Could you check a few things on this model? Use its own coordinates, in mm. A direction names the side the tool comes from. Give positions to 0.01 mm unless a question says otherwise; leave off trailing zeros. Order: outer loops, then holes, each group sorted by start corner. A loop starts at its lowest first (then second) coordinate and runs counter-clockwise, first axis right, second up. Notation, with made-up numbers: (-10, 72.25) -> (24, 72.25) arc R19 ccw to (24, 83.25) -> close; hole circle Ø8 at (-35.5, -7.75). An arc over 180 degrees is marked (long way). Write each question's results on one line, items separated by ' | '.
```python
from build123d import *

# Parameters (mm, degrees)
SKETCH1_R           = 3.6
BOSS_EXTRUDE2_DEPTH = 6
SKETCH4_R           = 4.250000009
BOSS_EXTRUDE3_DEPTH = 9
SKETCH7_R           = 2.1082
CUT_EXTRUDE3_DEPTH  = 5.6
SKETCH5_R           = 2.000000064
BOSS_EXTRUDE6_DEPTH = 9.156
FILLET3_R           = 0.7
SKETCH9_R           = 3.000000096
BOSS_EXTRUDE7_DEPTH = 5.6
FILLET4_R           = 0.7


with BuildPart() as part:
    # Sketch1 → Boss-Extrude2 (new body)
    with BuildSketch(Plane(origin=(0, 0, 0), x_dir=(1, 0, 0), z_dir=(0, 1, 0))):
        with Locations(Location((0, 0, 0), (0, 0, 270))):
            Circle(SKETCH1_R)
    extrude(amount=BOSS_EXTRUDE2_DEPTH)

    # Sketch4 → Boss-Extrude3 (add)
    with BuildSketch(Plane(origin=(0, 0, 0), x_dir=(1, 0, 0), z_dir=(0, 1, 0))):
        with Locations(Location((0, 0, 0), (0, 0, 270))):
            Circle(SKETCH4_R)
    extrude(amount=-BOSS_EXTRUDE3_DEPTH)

    # Sketch7 → Cut-Extrude3 (cut)
    with BuildSketch(Plane(origin=(0, 6, 0), x_dir=(1, 0, 0), z_dir=(0, 1, 0))):
        with Locations(Location((0, 0, 0), (0, 0, 270))):
            Circle(SKETCH7_R)
    extrude(amount=-CUT_EXTRUDE3_DEPTH, mode=Mode.SUBTRACT)

    # Sketch5 → Boss-Extrude6 (add)
    with BuildSketch(Plane(origin=(0, 0, 0), x_dir=(1, 0, 0), z_dir=(0, 1, 0))):
        with Locations(Location((0, 0, 0), (0, 0, 270))):
            Circle(SKETCH5_R)
    extrude(amount=BOSS_EXTRUDE6_DEPTH)

    # Fillet3
    fillet3_edges = [part.edges().sort_by_distance(p)[0] for p in [
        (0, 6, -2.1082),
        (0, 6, -3.6),
    ]]
    fillet(fillet3_edges, radius=FILLET3_R)

    # Sketch9 → Boss-Extrude7 (add)
    with BuildSketch(Plane(origin=(0, 9.156, 0), x_dir=(1, 0, 0), z_dir=(0, 1, 0))):
        with Locations(Location((0, 0, 0), (0, 0, 270))):
            Circle(SKETCH9_R)
    extrude(amount=BOSS_EXTRUDE7_DEPTH)

    # Fillet4
    fillet4_edges = [part.edges().sort_by_distance(p)[0] for p in [
        (0, 14.756, -3.000000096),
    ]]
    fillet(fillet4_edges, radius=FILLET4_R)


solid = part.part
```
Q1. Suppose I cut it at A-A on x = 0. Please give me the cut outline in (y, z), and give its area (3 significant figures).
Here are the results:
outline: (-9, -4.25) -> (0, -4.25) -> (0, -3.6) -> (5.3, -3.6) arc R0.7 ccw to (6, -2.9) -> (6, -2.81) arc R0.7 ccw to (5.3, -2.11) -> (0.4, -2.11) -> (0.4, -2) -> (9.16, -2) -> (9.16, -3) -> (14.06, -3) arc R0.7 ccw to (14.76, -2.3) -> (14.76, 2.3) arc R0.7 ccw to (14.06, 3) -> (9.16, 3) -> (9.16, 2) -> (0.4, 2) -> (0.4, 2.11) -> (5.3, 2.11) arc R0.7 ccw to (6, 2.81) -> (6, 2.9) arc R0.7 ccw to (5.3, 3.6) -> (0, 3.6) -> (0, 4.25) -> (-9, 4.25) -> close | area: 164 mm²
Q2. Suppose I cut it at D-D on y = 7.5. Please give me the cut outline in (x, z).
Here are the results:
outline: circle Ø4 at (0, 0)
Q3. I need wall thicknesses on line 1 along X through (y, z) = (-4, 2.25); line 2 along Y through (x, z) = (-2.75, 0.5); line 3 along Z through (x, y) = (0.75, 13). Which ranges of each line are inside material? Lowest first, please.
Here are the results:
line 1: x = -3.61 to 3.61 | line 2: y = -9 to 6, 9.16 to 14.55 | line 3: z = -2.9 to 2.9
Q4. Suppose I cut it at B-B on z = 0. Please give me the cut outline in (x, y), and give its area (3 significant figures).
Here are the results:
outline: (-4.25, -9) -> (4.25, -9) -> (4.25, 0) -> (3.6, 0) -> (3.6, 5.3) arc R0.7 ccw to (2.9, 6) -> (2.81, 6) arc R0.7 ccw to (2.11, 5.3) -> (2.11, 0.4) -> (2, 0.4) -> (2, 9.16) -> (3, 9.16) -> (3, 14.06) arc R0.7 ccw to (2.3, 14.76) -> (-2.3, 14.76) arc R0.7 ccw to (-3, 14.06) -> (-3, 9.16) -> (-2, 9.16) -> (-2, 0.4) -> (-2.11, 0.4) -> (-2.11, 5.3) arc R0.7 ccw to (-2.81, 6) -> (-2.9, 6) arc R0.7 ccw to (-3.6, 5.3) -> (-3.6, 0) -> (-4.25, 0) -> close | area: 164 mm²
Q5. I'm going to push flat-ended pins straight in: pin 1 Ø4 at (y, z) = (10.5, -3) entering from +X; pin 2 Ø1 at (x, z) = (2, 2.5) entering from +Y; pin 3 Ø4 at (x, y) = (-2, 8) entering from -Z. Where does each tip first touch, or does it pass through?
Here are the results:
pin 1: stops at x = 2.83 | pin 2: stops at y = 14.63 | pin 3: stops at z = -2.98
Q6. Suppose I cut it at C-C on y = -4.5. Please give me the cut outline in (x, z).
Here are the results:
outline: circle Ø8.5 at (0, 0)
Q7. For faces 1 (the cylindrical face through (-2.93, 11.57, -0.65)), 2 (the flat face through (-2, 9.156, 1)), 3 (the flat face through (0, 14.756, 0)), which set-ups out of +Z, -Z, +X, -X, +Y, -Y let a thin tool reach every point of the face, with its end or its side?
Here are the results:
face 1: +Y | face 2: none | face 3: +Z, -Z, +X, -X, +Y
